Check sheet for the modelled part. Datum: model origin and axes. Units: mm. A direction names the side the tool comes from. Coordinates: 2 decimals unless noted, no trailing zeros. Order: outer loops, then holes, each group sorted by start corner. A loop starts at its lowest first (then second) coordinate and runs counter-clockwise, first axis right, second up.
1. Gauge pin test, flat ends, axial feed: pin 1 Ø3 at (x, y) = (21, 16) entering from +Z; pin 2 Ø2 at (x, y) = (34.5, 11.5) entering from -Z; pin 3 Ø4 at (x, z) = (-3, 18) entering from -Y. Record the tip position at first contact, or that the pin passes through.
2. Cross-section at B-B (y = 18.5). Enter the section's corners in (x, z), then the cut area to 3 significant figures.
3. Cross-section at C-C (x = 26.5). Enter the section's corners in (y, z), then the cut area to 3 significant figures.
4. Cross-section at D-D (x = -4.5). Enter the section's corners in (y, z), then the cut area to 3 significant figures.
5. Set-up check for faces 1 (the flat face through (53.83, 24.5, 4.44)), 2 (the flat face through (10, 14, 19)): record each of +Z, -Z, +X, -X, +Y, -Y from which the full face is reachable in a straight line by a thin tool's end or side.
6. Thickness scan on line 1 (Z direction, x = 13.5, y = 26); line 2 (X direction, y = 21, z = 26); line 3 (X direction, y = 6, z = 28.25). Record the ranges inside material, lowest first.
```python
from build123d import *

# Parameters (mm, degrees)
F1_DEPTH = 9
F3_DEPTH = 21


with BuildPart() as f1:
    # F0 (on Top) → F1 (new body)
    with BuildSketch(Plane.XY):
        with BuildLine():
            ThreePointArc((0, 27.71285), (-13.856425, 13.856425), (0, 0))
            Line((0, 0), (49.899384, 0))
            Line((49.899384, 0), (55.913314, 5.932663))
            Line((55.913314, 5.932663), (55.913314, 21.37384))
            Line((55.913314, 21.37384), (51.687304, 27.71285))
            Line((51.687304, 27.71285), (0, 27.71285))
        make_face()
    extrude(amount=F1_DEPTH)

    # F2 (on face) → F3 (join)
    with BuildSketch(Plane.XY.offset(9)):
        with BuildLine():
            Line((10, 0), (10, 27.71285))
            Line((10, 27.71285), (0, 27.71285))
            ThreePointArc((0, 27.71285), (-13.856425, 13.856425), (0, 0))
            Line((0, 0), (10, 0))
        make_face()
    extrude(amount=F3_DEPTH)


solid = f1.part
```
Data:
1. pin 1: stops at z = 9
1. pin 2: stops at z = 0
1. pin 3: stops at y = 0.04
2. outline: (-13.06, 0) - (55.91, 0) - (55.91, 9) - (10, 9) - (10, 30) - (-13.06, 30) - close
2. area: 1,100 mm2
3. outline: (0, 0) - (27.71, 0) - (27.71, 9) - (0, 9) - close
3. area: 249 mm2
4. outline: (0.75, 0) - (26.96, 0) - (26.96, 30) - (0.75, 30) - close
4. area: 786 mm2
5. face 1: +Z, -Z, +X, +Y
5. face 2: +Z, +X, +Y, -Y
6. line 1: z = 0 to 9
6. line 2: x = -11.87 to 10
6. line 3: x = -11.41 to 10
